Autodesk Inventor part; units mm, degrees
ref_plane "Plano de trabajo3" through (185, 53, 51.5) normal (1, 0, 0) x (0, 0, -1)
ref_plane "Plano de trabajo4" through (125.2094, 54.5, 50) normal (1, 0, 0) x (0, 0, -1)
ref_plane "Plano de trabajo5" through (145.2094, 54.5, 50) normal (1, 0, 0) x (0, 0, -1)
ref_plane "Plano de trabajo3" through (185, 53, 51.5) normal (1, 0, 0) x (0, 0, -1)
ref_plane "Plano de trabajo4" through (125.2094, 54.5, 50) normal (1, 0, 0) x (0, 0, -1)
sketch "Boceto3" plane through (125.2094, 54.5, 50) normal (1, 0, 0) x (0, 0, -1)
  circle A0 centre (0, 0) radius 30
  circle A1 centre (0, 0) radius 5
  point P0 (50, -54.5)
  dimension "d5" = 60
  dimension "d9" = 10
extrude "Extrusión1" add sketch "Boceto3" along normal blind 40 contours A0 | A1
shell "Vaciado1" thickness 1 removed faces 2 at (125.2094, 56.8932, 44.7392) at (165.2094, 56.8932, 44.7392)
sketch "Boceto4" plane through (165.2094, 54.5, 50) normal (1, 0, 0) x (0, 0, -1)
  circle A0 centre (0, 0) radius 9
  circle A1 centre (0, 0) radius 4.1
  point P0 (50, -54.5)
  dimension "d10" = 18
  dimension "d11" = 8.2
extrude "Extrusión2" add sketch "Boceto4" against normal blind 40
sketch "Boceto5" plane through (165.2094, 54.5, 50) normal (1, 0, 0) x (0, 0, -1)
  line L0 (0, 0) -> (-4.1, 0)
  circle A0 centre (0, 0) radius 4.1
  line L1 (-4.1, 0) -> (-7.1, 0)
  line L2 (-1.1, -2.75) -> (-7.1, -2.75)
  line L3 (-7.1, -2.75) -> (-7.1, 2.75)
  line L4 (-7.1, 2.75) -> (-1.1, 2.75)
  line L5 (-1.1, 2.75) -> (-1.1, -2.75)
  line L6 (-1.1, -2.75) -> (-7.1, 2.75) construction
  line L7 (-7.1, -2.75) -> (-1.1, 2.75) construction
  point P0 (50, -54.5)
  point P1 (-3.041, -2.75)
  point P2 (-3.041, 2.75)
  dimension "d14" = 3
  dimension "d15" = 5.5
extrude "Extrusión3" cut sketch "Boceto5" against normal blind 5.5 contours L1 L3 L4 A0 | A0 L2 L3 L1
sketch "Boceto6" plane through (165.2094, 51.75, 57.1) normal (0, 0, -1) x (-1, 0, 0)
  line L0 (0, 0) -> (0, 5.5)
  line L1 (0, 0) -> (5.5, 0)
  line L2 (5.5, 0) -> (5.5, 5.5)
  line L3 (0, 5.5) -> (5.5, 5.5)
  line L4 (5.5, 0) -> (5.5, 5.5)
  line L5 (5.5, 5.5) -> (0, 0)
  circle A0 centre (2.75, 2.75) radius 1.5
  point P0 (165.2094, -51.75)
  dimension "d18" = 3
hole "Agujero1" at (162.4594, 54.5, 57.1) direction (0, 0, 1) diameter 3 depth 3.7 tip angle 118
ref_plane "Plano de trabajo5" through (145.2094, 54.5, 50) normal (1, 0, 0) x (0, 0, -1)
ref_plane "Plano de trabajo6" through (0, 0, 80) normal (0, 0, 1) x (1, 0, 0)
sketch "Boceto7" plane through (0, 0, 80) normal (0, 0, 1) x (1, 0, 0)
  line L0 (162.4594, 56) -> (162.4594, 53)
  circle A0 centre (162.4594, 54.5) radius 3.5
  point P0 (0, 0)
  dimension "d27" = 7
extrude "Extrusión4" cut sketch "Boceto7" against normal blind 5.5
mirror "Simetría2" about plane through (145.2094, 54.5, 50) normal (1, 0, 0) of "Extrusión4", "Agujero1", "Extrusión3"
sketch "Boceto10" plane through (165.2094, 54.5, 50) normal (1, 0, 0) x (0, 0, -1)
  line L0 (20.5061, -21.9203) -> (21.9203, -20.5061)
  line L1 (21.9203, -20.5061) -> (-20.5061, 21.9203)
  line L2 (-20.5061, 21.9203) -> (-21.9203, 20.5061)
  line L3 (-21.9203, 20.5061) -> (20.5061, -21.9203)
  line L4 (20.5061, -21.9203) -> (-20.5061, 21.9203) construction
  line L5 (21.9203, -20.5061) -> (-21.9203, 20.5061) construction
  line L6 (21.9203, 20.5061) -> (20.5061, 21.9203)
  line L7 (20.5061, 21.9203) -> (-21.9203, -20.5061)
  line L8 (-21.9203, -20.5061) -> (-20.5061, -21.9203)
  line L9 (-20.5061, -21.9203) -> (21.9203, 20.5061)
  line L10 (21.9203, 20.5061) -> (-21.9203, -20.5061) construction
  line L11 (20.5061, 21.9203) -> (-20.5061, -21.9203) construction
  line L12 (-3.041, -2.75) -> (-7.1, -2.75)
  line L13 (-7.1, -2.75) -> (-7.1, 2.75)
  line L14 (-7.1, 2.75) -> (-3.041, 2.75)
  arc A0 (-3.041, -2.75) -> (-3.041, 2.75) centre (0, 0) ccw
  circle A1 centre (0, 0) radius 9
  circle A2 centre (0, 0) radius 9
  point P0 (50, -54.5)
  point P1 (0, 0)
  point P2 (2.1045, 3.5187)
  point P3 (3.5187, 2.1045)
  point P4 (-2.1045, -3.5187)
  point P5 (-4.1642, -2.75)
  point P6 (-4.1642, 2.75)
  point P7 (-2.1045, 3.5187)
  point P8 (3.5187, -2.1045)
  point P9 (2.1045, -3.5187)
  dimension "d30" = 2
  dimension "d31" = 60
  dimension "d32" = 2
  dimension "d33" = 60
extrude "Extrusión5" add sketch "Boceto10" against normal blind 40 contours L3 A1 L1 L0 | L3 A0 L1 A1 | A1 L7 L12 A0 L9 | L9 L8 L7 A1 | A0 L7 A1 L9 | A1 L7 L6 L9 | A1 L1 A0 L14 L3 | L3 L2 L1 A1
properties part number "Rampa"
Read the model definition and answer for the solid it produces. Units are mm, in the model's axes. A direction names the side the tool comes from. Coordinates: 2 decimals unless noted, no trailing zeros. Order: outer loops, then holes, each group sorted by start corner. A loop starts at its lowest first (then second) coordinate and runs counter-clockwise, first axis right, second up. Notation, with made-up numbers: (1.25, 86) -> (28.25, 86) arc R37 cw to (28.25, 124) -> close; hole circle Ø2 at (45, 61). An arc over 180 degrees is marked (long way). Answer as a JSON object with one key per item and string values.
1) Consider line 1 along Z through (x, y) = (149.5, 61.5); line 2 along Y through (x, z) = (138, 49); line 3 along Y through (x, z) = (135, 63). Determine where each line is inside the solid, lowest interval first. Write a range as from..to.
Model answer:
{"line 1": "z = 20.83..21.86, 41.59..58.41, 78.14..79.17", "line 2": "y = 24.52..25.52, 45.56..50.52, 58.48..63.44, 83.48..84.48", "line 3": "y = 27.46..28.58, 40.09..42.91, 66.09..68.91, 80.42..81.54"}
2) The mould has two halves that part along Y. Classify faces 1 (the face through (128, 51.75, 55)), 2 (the face through (165.209, 59, 50)), 3 (the face through (144.9, 84.5, 50.3)), 4 (the face through (145.489, 33.277, 28.797)): released by +Y, released by -Y, zero draft, split by the parting line, or undercut.
Model answer:
{"face 1": "undercut", "face 2": "zero draft", "face 3": "released by +Y", "face 4": "released by -Y"}
3) A cutting plane is placed at C-C, the plane x = 149. State how many separate pieces and enclosed holes the cut face has, plus the area to 3 significant figures.
Model answer:
{"separate pieces": "1", "enclosed holes": "5", "area": "547 mm²"}
4) A cutting plane is placed at A-A, the plane y = 54.5. Determine the outline of the cut face in (x, z), plus the area to 3 significant figures.
Model answer:
{"outline": "(125.21, 20) -> (165.21, 20) -> (165.21, 21) -> (125.21, 21) -> close; (125.21, 41) -> (165.21, 41) -> (165.21, 45.9) -> (125.21, 45.9) -> close; (125.21, 57.1) -> (126.46, 57.1) -> (126.46, 59) -> (125.21, 59) -> close; (129.46, 57.1) -> (130.71, 57.1) -> (130.71, 54.1) -> (159.71, 54.1) -> (159.71, 57.1) -> (160.96, 57.1) -> (160.96, 59) -> (129.46, 59) -> close; (131.46, 79) -> (158.96, 79) -> (158.96, 80) -> (131.46, 80) -> close; (163.96, 57.1) -> (165.21, 57.1) -> (165.21, 59) -> (163.96, 59) -> close", "area": "415 mm²"}
5) A cutting plane is placed at B-B, the plane z = 50. Determine the outline of the cut face in (x, y), plus the area to 3 significant figures.
Model answer:
{"outline": "(125.21, 24.5) -> (165.21, 24.5) -> (165.21, 25.5) -> (125.21, 25.5) -> close; (125.21, 45.5) -> (165.21, 45.5) -> (165.21, 50.4) -> (125.21, 50.4) -> close; (125.21, 58.6) -> (165.21, 58.6) -> (165.21, 63.5) -> (125.21, 63.5) -> close; (125.21, 83.5) -> (165.21, 83.5) -> (165.21, 84.5) -> (125.21, 84.5) -> close", "area": "472 mm²"}
6) A tool of negligible diameter and unlimited length cuts with its end or side. For faces 5 (the face through (145.489, 67.301, 64.216)), 6 (the face through (131.457, 54.379, 79.403)), 7 (the face through (161, 53, 57.1)), from which of +Z, -Z, +X, -X, +Y, -Y can it reach the whole face along a straight path? Write none if from no direction.
Model answer:
{"face 5": "+X, -X", "face 6": "+Z", "face 7": "+X"}
7) Each of these flat-tipped pins is pushed along its axis until it touches: pin 1 (5 mm diameter, centred on x = 136.5, z = 72.5, fed in from +Y); pin 2 (4 mm diameter, centred on x = 127.96, y = 54.5, fed in from -Z); pin 3 (1 mm diameter, centred on x = 153.5, y = 62, fed in from -Z); pin 4 (8 mm diameter, centred on x = 162.46, y = 54.5, fed in from +Z). Where does it stop, or does it pass through?
Model answer:
{"pin 1": "stops at y = 76.86", "pin 2": "stops at z = 20", "pin 3": "stops at z = 20.83", "pin 4": "stops at z = 80"}
8) A cutting plane is placed at D-D, the plane y = 38. Determine the outline of the cut face in (x, z).
Model answer:
{"outline": "(125.21, 24.95) -> (165.21, 24.95) -> (165.21, 26.15) -> (125.21, 26.15) -> close; (125.21, 32.09) -> (165.21, 32.09) -> (165.21, 34.91) -> (125.21, 34.91) -> close; (125.21, 65.09) -> (165.21, 65.09) -> (165.21, 67.91) -> (125.21, 67.91) -> close; (125.21, 73.85) -> (165.21, 73.85) -> (165.21, 75.05) -> (125.21, 75.05) -> close"}
